from build123d import *

# Parameters (mm, degrees)
F0_W     = 33.5
F0_H     = 37
F1_DEPTH = 10
F3_DEPTH = 37
F4_DEPTH = 10
F6_DEPTH = 15
F7_R     = 1


with BuildPart() as f1:
    # F0 (on Top) → F1 (new body)
    with BuildSketch(Plane.XY):
        Rectangle(F0_W, F0_H)
    extrude(amount=F1_DEPTH)

    # F2 (on face) → F3 (cut, through all)
    with BuildSketch(Plane.XZ.offset(18.5)):
        Polygon((-13.5, 7.5), (-15, 7.5), (-15, 5.4), (-14.5, 5), (-15, 4.6), (-15, 2.5), (-13.5, 2.5), (-13.1, 3), (-12.7, 2.5), (-1.9, 2.5), (-0.4, 2.5), (0, 3), (0.4, 2.5), (11.2, 2.5), (12.7, 2.5), (13.1, 3), (13.5, 2.5), (15, 2.5), (15, 4.6), (14.5, 5), (15, 5.4), (15, 7.5), (13.5, 7.5), (13.1, 7), (12.7, 7.5), (0.4, 7.5), (0, 7), (-0.4, 7.5), (-12.7, 7.5), (-13.1, 7), align=None)
    extrude(amount=-F3_DEPTH, mode=Mode.SUBTRACT)

    # F0 (on Top) → F4 (join)
    with BuildSketch(Plane.XY):
        Polygon((-5, 38.5), (-16.75, 18.5), (16.75, 18.5), (5, 38.5), align=None)
    extrude(amount=F4_DEPTH)

    # F5 (on face) → F6 (cut)
    with BuildSketch(Plane(origin=(0, 38.5, 0), x_dir=(-1, 0, 0), z_dir=(0, 1, 0))):
        Polygon((-3.2, 6.8475208614), (-3.2, 3.1524791386), (0, 1.3049582772), (3.2, 3.1524791386), (3.2, 6.8475208614), (0, 8.6950417228), align=None)
    extrude(amount=-F6_DEPTH, mode=Mode.SUBTRACT)

    # F7
    f7_edges = [f1.edges().sort_by_distance(p)[0] for p in [
        (-16.75, 0, 10),
        (0, -18.5, 10),
        (16.75, 0, 10),
        (10.875, 28.5, 10),
        (0, 38.5, 10),
        (-10.875, 28.5, 10),
        (-16.75, 0, 0),
        (0, -18.5, 0),
        (16.75, 0, 0),
        (10.875, 28.5, 0),
        (0, 38.5, 0),
        (-10.875, 28.5, 0),
        (-16.75, 18.5, 5),
        (-16.75, -18.5, 5),
        (-5, 38.5, 5),
        (16.75, 18.5, 5),
        (5, 38.5, 5),
        (16.75, -18.5, 5),
    ]]
    fillet(f7_edges, radius=F7_R)


solid = f1.part
Here's how the part is built. I have some questions about the finished solid (model axes, mm). A direction names the side the tool comes from. Give positions to 0.01 mm unless a question says otherwise; leave off trailing zeros. Order: outer loops, then holes, each group sorted by start corner. A loop starts at its lowest first (then second) coordinate and runs counter-clockwise, first axis right, second up. Notation, with made-up numbers: (-29, 10) -> (18, 10) arc R35 cw to (18, 47) -> close; hole circle Ø2 at (-11.5, 84.25). An arc over 180 degrees is marked (long way). One line per item, written item: value. Start each with the question number.
1. For faces 5 (the face through (-3.2, 31, 5)), 6 (the face through (-16.75, 0, 5)), 7 (the face through (6, 0, 2.5)), which set-ups out of +Z, -Z, +X, -X, +Y, -Y let a thin tool reach every point of the face, with its end or its side?
2. Imagine slicing it at A-A, the plane z = 4. List the corners of the cut face in (x, y) for me.
3. Will these pins go through, and if not, where does the flat tip stop? pin 1 Ø4 at (y, z) = (31, 5) entering from +X; pin 2 Ø4 at (y, z) = (32.5, 5.5) entering from -X; pin 3 Ø3 at (x, z) = (-1, 5.5) entering from +Y.
4. I need wall thicknesses on probe 1 along Z at (x, y) = (11.5, -10); probe 2 along X at (y, z) = (-6.5, 5.5); probe 3 along Y at (x, z) = (3.5, 3.25). Which ranges of each line are inside material? Lowest first, please. Write a range as from..to.
5. We'd pull the mould along X, two halves only. Please class faces 1 (the face through (0, 18.5, 5)), 2 (the face through (0, 4, 10)), 3 (the face through (-10.784, 28.091, 0.301)), 4 (the face through (10.6, 28.4, 9.7)): released by +X, released by -X, zero draft, split by the parting line, or undercut.
Values follow:
1. face 5: +Y
1. face 6: +Z, -Z, -X, +Y, -Y
1. face 7: -Y
2. outline: (-16.75, -17.5) arc R1 ccw to (-15.75, -18.5) -> (-15, -18.5) -> (-15, 18.5) -> (15, 18.5) -> (15, -18.5) -> (15.75, -18.5) arc R1 ccw to (16.75, -17.5) -> (16.75, 18.23) arc R1 ccw to (16.61, 18.73) -> (5.29, 38.01) arc R1 ccw to (4.43, 38.5) -> (3.2, 38.5) -> (3.2, 23.5) -> (-3.2, 23.5) -> (-3.2, 38.5) -> (-4.43, 38.5) arc R1 ccw to (-5.29, 38.01) -> (-16.61, 18.73) arc R1 ccw to (-16.75, 18.23) -> close
3. pin 1: stops at x = 10.58
3. pin 2: stops at x = -9.7
3. pin 3: stops at y = 23.5
4. probe 1: z = 0..2.5, 7.5..10
4. probe 2: x = -16.75..-15, 15..16.75
4. probe 3: y = 18.5..38.5
5. face 1: undercut
5. face 2: zero draft
5. face 3: released by -X
5. face 4: released by +X
